Here's how the part is built. I have some questions about the finished solid (model axes, mm). Round coordinates to 2 decimals unless told otherwise and drop trailing zeros. Order: outer loops, then holes, each group sorted by start corner. A loop starts at its lowest first (then second) coordinate and runs counter-clockwise, first axis right, second up. Notation, with made-up numbers: (39.5, 34.5) - (73.5, 34.5) arc R20 ccw to (73.5, 42.5) - close; hole circle Ø10 at (33.25, 42.5). An arc over 180 degrees is marked (long way). One line per item, written item: value.
Autodesk Inventor part; units mm, degrees
ref_plane "YZ Plane" through (0, 0, 0) normal (1, 0, 0) x (0, 1, 0)
ref_plane "XZ Plane" through (0, 0, 0) normal (0, 1, 0) x (-1, 0, 0)
ref_plane "XY Plane" through (0, 0, 0) normal (0, 0, 1) x (1, 0, 0)
sketch "Sketch1" plane through (0, 0, 0) normal (0, 1, 0) x (-1, 0, 0)
  line L0 (0, 0) -> (53.34, 0)
  line L1 (53.34, 0) -> (53.34, -107.95)
  line L2 (53.34, -107.95) -> (0, -107.95)
  line L3 (0, -107.95) -> (0, 0)
  point P0 (50.34, -5.5)
  point P1 (3.34, -5.5)
  point P2 (50.7579, -54.61)
  point P3 (2.8578, -53.34)
  point P4 (35.56, -105.41)
  point P5 (7.62, -105.41)
  dimension "d0" = 53.34
  dimension "d1" = 107.95
  dimension "d2" = 3
  dimension "d3" = 5.5
  dimension "d4" = 5.5
  dimension "d5" = 3.34
  dimension "d6" = 53.34
  dimension "d7" = 54.61
  dimension "d8" = 2.54
  dimension "d9" = 2.54
  dimension "d10" = 7.62
  dimension "d11" = 17.78
extrude "Extrusion1" add sketch "Sketch1" against normal blind 1.65
hole "Hole1" at (-50.34, 0, -5.5) at (-3.34, 0, -5.5) at (-50.7579, 0, -54.61) at (-2.8578, 0, -53.34) at (-35.56, 0, -105.41) at (-7.62, 0, -105.41) direction (0, -1, 0) diameter 3.2 end through all
sketch "Sketch2" plane through (0, 0, 0) normal (0, 1, 0) x (1, 0, 0)
  line L0 (-53.34, 0) -> (0, 0)
  line L1 (0, 0) -> (0, 107.95)
  circle A0 centre (-26.67, 23.67) radius 17.2
  line L2 (-26.67, 23.67) -> (-26.67, 130.1739)
  line L3 (-26.67, 23.67) -> (-67.3773, 47.1724)
  line L4 (-26.67, 23.67) -> (20.3348, 23.67) construction
  line L5 (-26.67, 23.67) -> (24.306, 53.101)
  line L6 (-26.67, 23.67) -> (32.192, 23.67) construction
  point P0 (-26.67, 40.87)
  point P1 (-11.7744, 32.27)
  point P2 (-26.67, 40.87)
  point P3 (-41.5656, 32.27)
  dimension "d21" = 23.67
  dimension "d22" = 26.67
  dimension "d23" = 34.4
  dimension "d24" = 150
  dimension "d25" = 30
hole "Hole2" at (-26.67, 0, -40.87) at (-11.7744, 0, -32.27) at (-41.5656, 0, -32.27) direction (0, -1, 0) diameter 2.58 end through all
properties part number "EChem Sensor Board Lower"
Q1. If we section it at A-A, the plane z = -105.41: Please give me the cut outline in (x, y).
Results list:
outline: (-53.34, -1.65) - (-37.16, -1.65) - (-37.16, 0) - (-53.34, 0) - close; (-33.96, -1.65) - (-9.22, -1.65) - (-9.22, 0) - (-33.96, 0) - close; (-6.02, -1.65) - (0, -1.65) - (0, 0) - (-6.02, 0) - close
Q2. If I drill on line 1 along X through (y, z) = (-0.7, -32.27); line 2 along Z through (x, y) = (-26.67, -0.7); line 3 along Z through (x, y) = (-3.34, -1.25), over which ranges is the centre line in solid material (lowest first)?
Results list:
line 1: -53.34 to -42.86, -40.28 to -13.06, -10.48 to 0
line 2: -107.95 to -42.16, -39.58 to 0
line 3: -107.95 to -54.87, -51.81 to -7.1, -3.9 to 0
Q3. If we section it at C-C, the plane x = -7.62: Please give me the cut outline in (y, z).
Results list:
outline: (-1.65, -107.95) - (0, -107.95) - (0, -107.01) - (-1.65, -107.01) - close; (-1.65, -103.81) - (0, -103.81) - (0, 0) - (-1.65, 0) - close
Q4. If we section it at B-B, the plane x = -26.67: Please give me the cut outline in (y, z).
Results list:
outline: (-1.65, -107.95) - (0, -107.95) - (0, -42.16) - (-1.65, -42.16) - close; (-1.65, -39.58) - (0, -39.58) - (0, 0) - (-1.65, 0) - close
Q5. We'd pull the mould along Z, two halves only. Please class faces 1 (the cylindrical face through (-27.06, -0.84, -39.64)), 2 (the flat face through (-26, 0, -53)): released by +Z, released by -Z, zero draft, split by the parting line, or undercut.
Results list:
face 1: undercut
face 2: zero draft
Q6. Will this pin go through, and if not, where does the flat tip stop? pin 1 (8 mm diameter, centred on x = -19, z = -32.5, fed in from +Y).
Results list:
pin 1: y = 0
